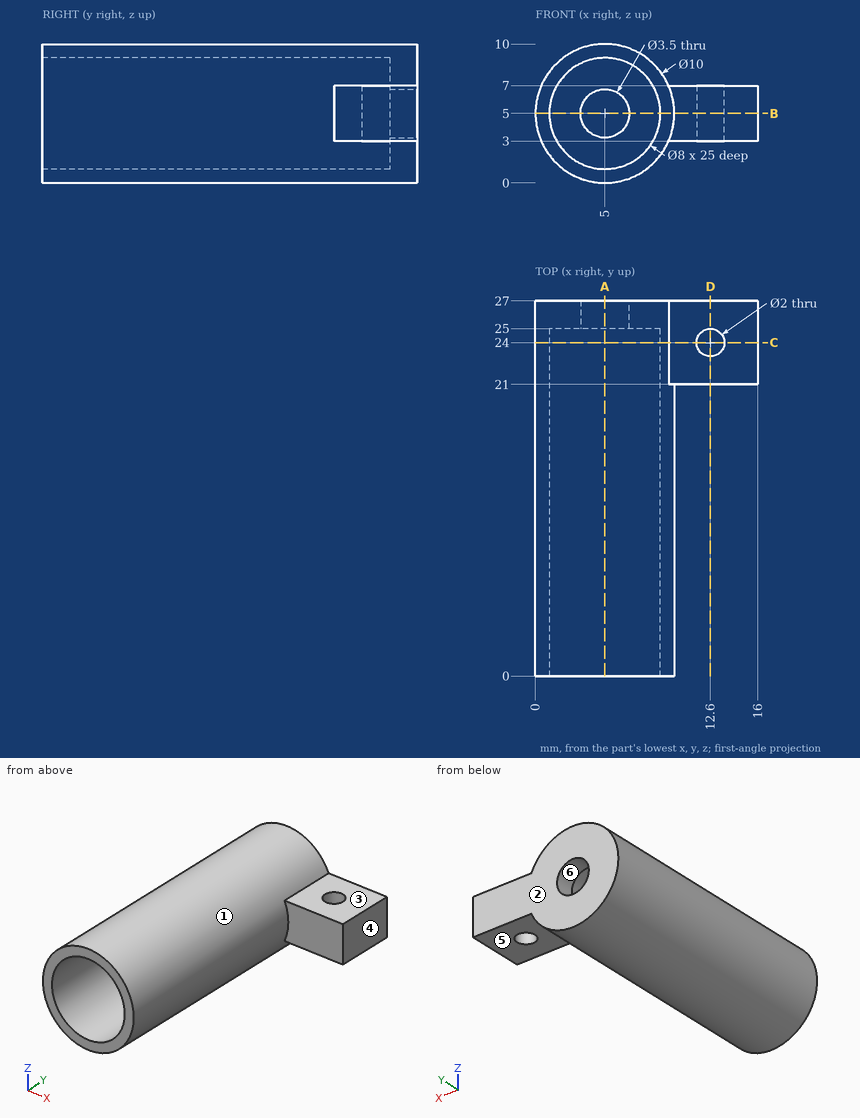
Answer from the drawing. Dimensions are ordinates in mm from the lowest x, y and z of the part. A direction names the side the tool comes from. Give positions to 0.01 mm unless a question says otherwise; leave off trailing zeros. Write each loop counter-clockwise with the first axis right and the second up, starting at its lowest first coordinate (ties: lowest second). Pieces come first, ordered by that corner, then holes. Notation, with made-up numbers: (-39, -23.75) - (-19, -23.75) arc R32 cw to (-19, 2.25) - close; hole circle Ø3 at (52, 69). An arc over 180 degrees is marked (long way). Answer in a Markdown table with one row per item. Add a question column.
Item 1: Find the intervals of material crossed by L1, parallel to Z at x = 5, y = 13.5; L2, parallel to Y at x = 12.5, z = 5.75; L3, parallel to Z at x = 5, y = 26.1, in increasing order.
Item 2: Section C-C, the plane y = 24 is taken. Write down the section's boundary in (x, z).
Item 3: Flat-ended cylindrical pins translate along their axes: P1, Ø3, axis at x = 12.5, y = 23.5, coming from the +Z side; P2, Ø2.5, axis at x = 12.6, y = 24, coming from the -Z side; P3, Ø2.5, axis at x = 6, z = 3.5, coming from the -Y side. Find the tip coordinate at first contact, or state that the pin passes through.
Item 4: Section D-D, the plane x = 12.6 is taken. Write down the section's boundary in (y, z).
Item 5: Determine the mould class of the marked faces 4, 5 and 6 for opening direction Z: pulls with the +Z half, pulls with the -Z half, needs draft (parallel to the pull), parting line crosses it, or undercut.
Item 6: A tool of negligible diameter and unlimited length cuts with its end or side. For the marked faces 1, 2 and 3, from which of +Z, -Z, +X, -X, +Y, -Y can it reach the whole face along a straight path? Write none if from no direction.
Item 7: Section B-B, the plane z = 5 is taken. Write down the section's boundary in (x, y), and give its area (3 significant figures).
Item 8: Section A-A, the plane x = 5 is taken. Write down the section's boundary in (y, z), and give its area (3 significant figures).
Recorded:
| question | item | result |
|---|---|---|
| 1 | L1 | z = 0 to 1, 9 to 10 |
| 1 | L2 | y = 21 to 23.01, 24.99 to 27 |
| 1 | L3 | z = 0 to 3.25, 6.75 to 10 |
| 2 | outline | (9.58, 3) - (11.6, 3) - (11.6, 7) - (9.58, 7) arc R5 ccw (long way) to start; (13.6, 3) - (16, 3) - (16, 7) - (13.6, 7) - close; hole circle Ø8 at (5, 5) |
| 3 | P1 | stops at z = 7 |
| 3 | P2 | stops at z = 3 |
| 3 | P3 | stops at y = 25 |
| 4 | outline | (21, 3) - (23, 3) - (23, 7) - (21, 7) - close; (25, 3) - (27, 3) - (27, 7) - (25, 7) - close |
| 5 | face 4 | needs draft |
| 5 | face 5 | pulls with the -Z half |
| 5 | face 6 | undercut |
| 6 | face 1 | -Y |
| 6 | face 2 | +Z, -Z, +X, -X, +Y |
| 6 | face 3 | +Z, +X, +Y, -Y |
| 7 | outline | (0, 0) - (1, 0) - (1, 25) - (3.25, 25) - (3.25, 27) - (0, 27) - close; (6.75, 25) - (9, 25) - (9, 0) - (10, 0) - (10, 21) - (16, 21) - (16, 27) - (6.75, 27) - close; hole circle Ø2 at (12.6, 24) |
| 7 | area | 95.9 mm2 |
| 8 | outline | (0, 0) - (27, 0) - (27, 3.25) - (25, 3.25) - (25, 1) - (0, 1) - close; (0, 9) - (25, 9) - (25, 6.75) - (27, 6.75) - (27, 10) - (0, 10) - close |
| 8 | area | 63.0 mm2 |
